For this review, take the finished solid that the model builds, in its own axes (mm). A direction names the side the tool comes from. Round coordinates to 2 decimals unless told otherwise and drop trailing zeros. Write each loop counter-clockwise with the first axis right and the second up, starting at its lowest first coordinate (ties: lowest second). Pieces come first, ordered by that corner, then holes.
from build123d import *

# Parameters (mm, degrees)
SKETCH_1_R      = 1.5
SKETCH_1_R_2    = 0.75
SKETCH_1_W      = 23
SKETCH_1_H      = 12
EXTRUDE_3_DEPTH = 3


with BuildPart() as part:
    # 草图1 → 凸台-拉伸3 (new body)
    with BuildSketch(Plane(origin=(0, 0, 0), x_dir=(1, 0, 0), z_dir=(0, 1, 0))):
        Polygon((-15.016304348, 6.130434783), (-15.016304348, 15.130434783), (-13.516304348, 15.130434783), (-13.516304348, 12.130434783), (-10.516304348, 12.130434783), (-10.516304348, 15.065217391), (19.483695652, 15.065217391), (19.483695652, 11.065217391), (22.483695652, 11.065217391), (22.483695652, 1.065217391), (19.483695652, 1.065217391), (19.483695652, -2.934782609), (-10.516304348, -2.934782609), (-10.516304348, 0), (-13.516304348, 0), (-13.516304348, -3), (-15.016304348, -3), (-15.016304348, 6), align=None)
        with Locations(Location((20.926676996, 6.065217391, 0), (0, 0, 270))):
            Circle(SKETCH_1_R, mode=Mode.SUBTRACT)
        with Locations(Location((-10.916304348, 6.065217391, 0), (0, 0, 270))):
            Circle(SKETCH_1_R_2, mode=Mode.SUBTRACT)
        with Locations(Location((16.583695652, 6.065217391, 0), (0, 0, 270))):
            Circle(SKETCH_1_R_2, mode=Mode.SUBTRACT)
        with Locations((2.833695652, 6.065217391)):
            Rectangle(SKETCH_1_W, SKETCH_1_H, mode=Mode.SUBTRACT)
    extrude(amount=EXTRUDE_3_DEPTH)


solid = part.part
(1) For faces 4 (the face through (21, 1, -11.065)), 5 (the face through (-13.516, 1, 1)), 6 (the face through (-12, 1, -12.13)), 7 (the face through (5, 1, 2.935)), 8 (the face through (-8.666, 1, -6)), list the 3-axis set-ups (+Z, -Z, +X, -X, +Y, -Y) from which the entire face can be reached by the end or side of a thin tool; tool diameter is ignored.
Geometry check:
face 4: -Z, +X, +Y, -Y
face 5: +Z, +Y, -Y
face 6: -Z, +Y, -Y
face 7: +Z, +X, +Y, -Y
face 8: +Y, -Y
(2) Mouldability with a two-part tool opening along X and no side actions: class faces 1 (the face through (-15.016, 1, -6)), 2 (the face through (4, 3, -12.24)), 3 (the face through (14.334, 1, -6)) as pulls with the +X half, pulls with the -X half, needs draft (parallel to the pull), parting line crosses it, or undercut.
Geometry check:
face 1: pulls with the -X half
face 2: needs draft
face 3: undercut
(3) For line 1 along Z through (x, y) = (-8.5, 0.4); line 2 along X through (y, z) = (1.7, -2.5); line 3 along X through (y, z) = (2.4, -11.75), list the stretches that pass through material, from the lowest coordinate up.
Geometry check:
line 1: z = -15.07 to -12.07, -0.07 to 2.93
line 2: x = -15.02 to -8.67, 14.33 to 22.48
line 3: x = -15.02 to -8.67, 14.33 to 19.48
(4) For pin 1 Ø0.9 at (x, y) = (2.5, 2) entering from +Z; pin 2 Ø0.9 at (y, z) = (2, 1.5) entering from +X, all flat-tipped, find the tip position at first contact; note any pin that passes through.
Geometry check:
pin 1: stops at z = 2.93
pin 2: stops at x = 19.48
(5) We need section A-A, the plane z = 0.5. Give the boundary of the cut face in (x, y), and give its area (3 significant figures).
Geometry check:
outline: (-15.02, 0) - (-13.52, 0) - (-13.52, 3) - (-15.02, 3) - close; (-10.52, 0) - (19.48, 0) - (19.48, 3) - (-10.52, 3) - close
area: 94.5 mm2
(6) We need section C-C, the plane y = 1.75. Give the boundary of the cut face in (x, z), and give its area (3 significant figures).
Geometry check:
outline: (-15.02, -15.13) - (-13.52, -15.13) - (-13.52, -12.13) - (-10.52, -12.13) - (-10.52, -15.07) - (19.48, -15.07) - (19.48, -11.07) - (22.48, -11.07) - (22.48, -1.07) - (19.48, -1.07) - (19.48, 2.93) - (-10.52, 2.93) - (-10.52, 0) - (-13.52, 0) - (-13.52, 3) - (-15.02, 3) - close; hole circle Ø1.5 at (-10.92, -6.07); hole (-8.67, -12.07) - (14.33, -12.07) - (14.33, -0.07) - (-8.67, -0.07) - close; hole circle Ø1.5 at (16.58, -6.07); hole circle Ø3 at (20.93, -6.07)
area: 347 mm2
(7) We need section B-B, the plane x = -3.5. Give the boundary of the cut face in (y, z).
Geometry check:
outline: (0, -15.07) - (3, -15.07) - (3, -12.07) - (0, -12.07) - close; (0, -0.07) - (3, -0.07) - (3, 2.93) - (0, 2.93) - close
